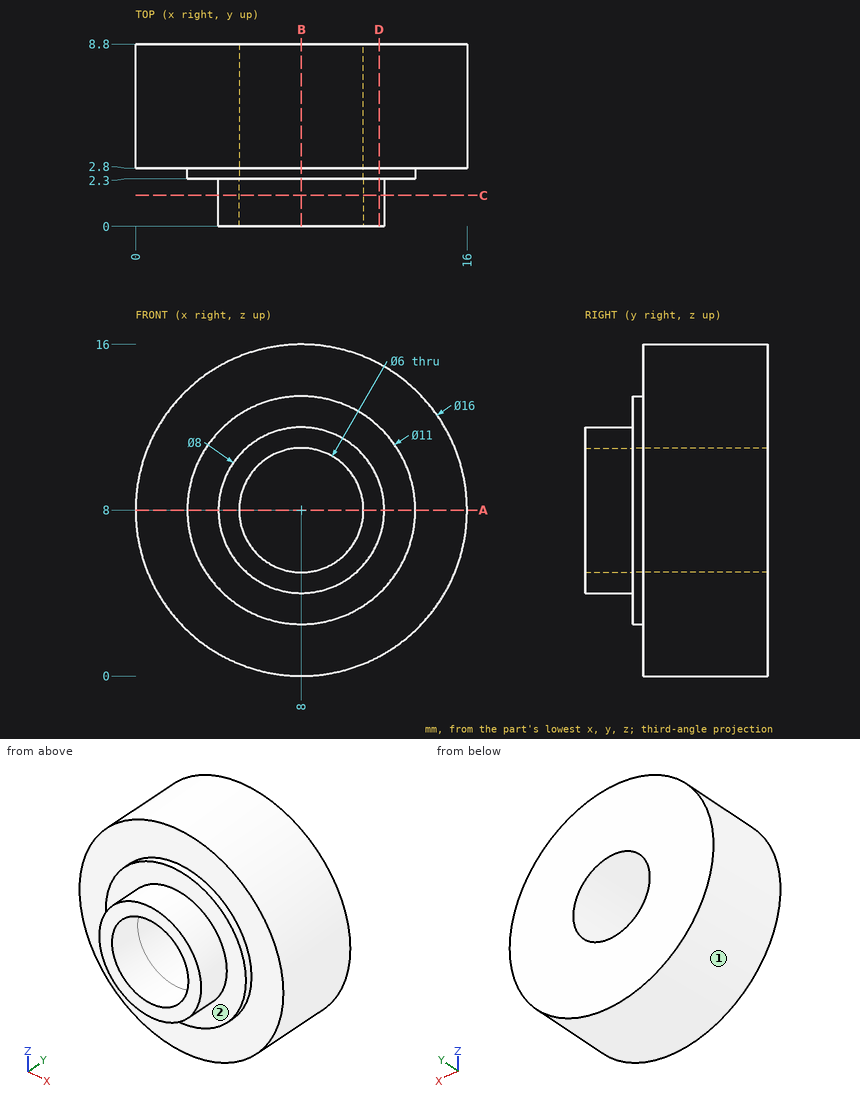
Design review of the part shown in the three views and the two pictorial views. Dimensions are in mm from the part's minimum x, y and z. A direction names the side the tool comes from. Coordinates: 2 decimals unless noted, no trailing zeros. Loops run counter-clockwise (first coordinate to the right, second up) from the corner with the lowest first, then second, coordinate; pieces in that order, holes last. Notation, with made-up numbers: (35, 45.5) -> (79, 45.5) arc R17 cw to (79, 53.5) -> close; hole circle Ø5 at (29.25, 60.25). An arc over 180 degrees is marked (long way). Answer as CSV lines item,"result".
Item 1: Take a section at C-C, the plane y = 1.5. State the section outline as (x, z) points.
Results below:
outline,"circle Ø8 at (8, 8); hole circle Ø6 at (8, 8)"
Item 2: Take a section at A-A, the plane z = 8. State the section outline as (x, y) points, and give its area (3 significant figures).
Results below:
outline,"(0, 2.8) -> (2.5, 2.8) -> (2.5, 2.3) -> (4, 2.3) -> (4, 0) -> (5, 0) -> (5, 8.8) -> (0, 8.8) -> close; (11, 0) -> (12, 0) -> (12, 2.3) -> (13.5, 2.3) -> (13.5, 2.8) -> (16, 2.8) -> (16, 8.8) -> (11, 8.8) -> close"
area,"67.1 mm2"
Item 3: Take a section at D-D, the plane x = 11.75. State the section outline as (y, z) points.
Results below:
outline,"(0, 6.61) -> (2.3, 6.61) -> (2.3, 3.98) -> (2.8, 3.98) -> (2.8, 0.93) -> (8.8, 0.93) -> (8.8, 15.07) -> (2.8, 15.07) -> (2.8, 12.02) -> (2.3, 12.02) -> (2.3, 9.39) -> (0, 9.39) -> close"
Item 4: Machinability: for the marked faces 1 and 2, which of the approach directions +Z, -Z, +X, -X, +Y, -Y give a long, thin tool a straight path to every point of the face, cutting with its end or side? Answer none if there is none.
Results below:
face 1,"+Y, -Y"
face 2,"-Y"
Item 5: For L1, parallel to Z at x = 8, y = 5.75; L2, parallel to Z at x = 8, y = 1.55; L3, parallel to Y at x = 2.5, z = 11.25, list the stretches that pass through material, from the lowest coordinate up.
Results below:
L1,"z = 0 to 5, 11 to 16"
L2,"z = 4 to 5, 11 to 12"
L3,"y = 2.8 to 8.8"
Item 6: Insertion check: pin 1 (5.5 mm diameter, centred on x = 8.5, z = 6, fed in from -Y); pin 2 (4 mm diameter, centred on y = 7.5, z = 2, fed in from +X); pin 3 (2 mm diameter, centred on y = 3, z = 11.5, fed in from -X); pin 4 (1 mm diameter, centred on x = 13.5, y = 1, fed in from -Z) (3 decimals). Each pin has a flat end and moves straight along its axis. Give the tip position at first contact, or say it passes through.
Results below:
pin 1,"stops at y = 0"
pin 2,"stops at x = 14.93"
pin 3,"stops at x = 0.4"
pin 4,"passes through"
Item 7: Take a section at B-B, the plane x = 8. State the section outline as (y, z) points, and give its area (3 significant figures).
Results below:
outline,"(0, 4) -> (2.3, 4) -> (2.3, 2.5) -> (2.8, 2.5) -> (2.8, 0) -> (8.8, 0) -> (8.8, 5) -> (0, 5) -> close; (0, 11) -> (8.8, 11) -> (8.8, 16) -> (2.8, 16) -> (2.8, 13.5) -> (2.3, 13.5) -> (2.3, 12) -> (0, 12) -> close"
area,"67.1 mm2"
